Drawing for the job (mm, zero at the part's lowest x, y, z). A direction names the side the tool comes from. Give positions to 0.01 mm unless a question says otherwise; leave off trailing zeros. Write each loop counter-clockwise with the first axis right and the second up, starting at its lowest first coordinate (ties: lowest second). Pieces come first, ordered by that corner, then holes. Notation, with made-up numbers: (35.25, -38) - (90.25, -38) arc R31 cw to (90.25, -7) - close; hole circle Ø1 at (78, -19.75). An arc over 180 degrees is marked (long way). Use CSV: the item, a comma, the result in double quotes.
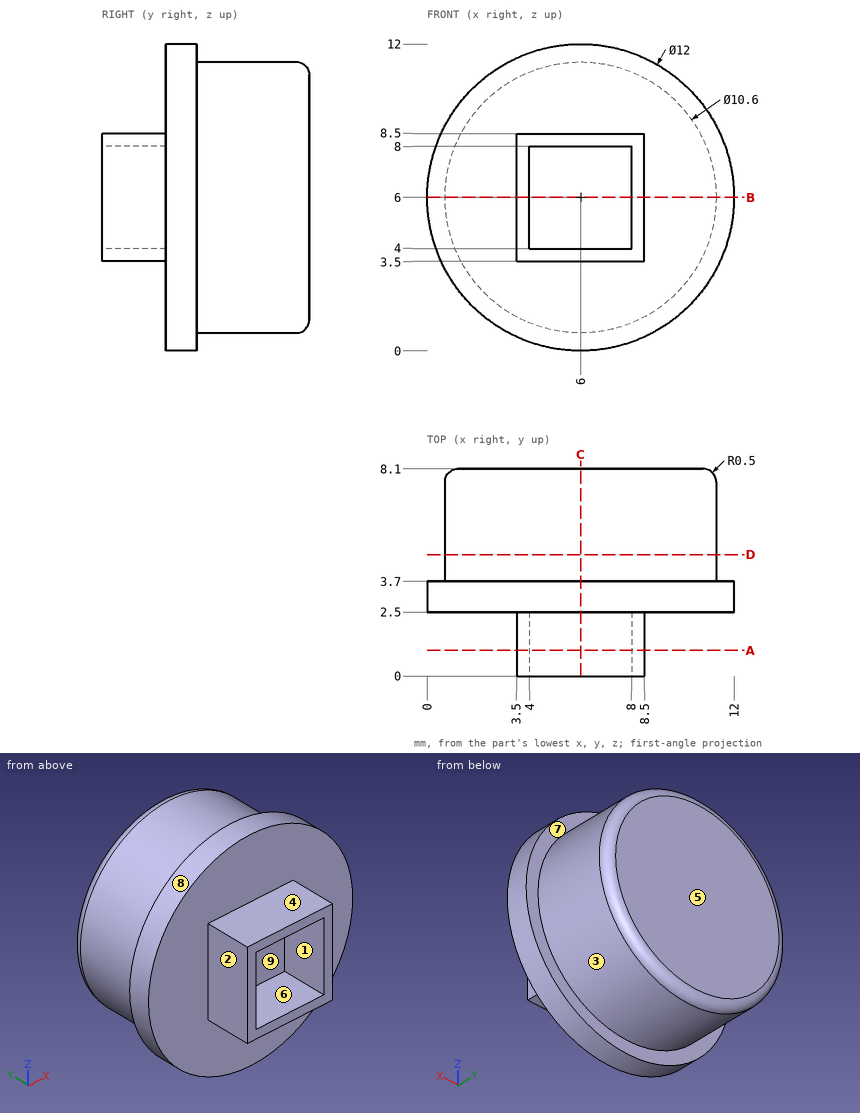
(1) Pull direction Z, two halves, no side cores. Call the marked faces 6, 7, 8 and 9: released by +Z, released by -Z, zero draft, split by the parting line, or undercut.
Checked values:
face 6,"undercut"
face 7,"zero draft"
face 8,"split by the parting line"
face 9,"undercut"
(2) Flat gauge pins, fed straight in: P1, Ø2, axis at x = 5, y = 2, coming from the -Z side; P2, Ø0.8, axis at x = 6, y = 1, coming from the +Z side; P3, Ø2, axis at y = 0.5, z = 5.5, coming from the +X side. Where does each tip first touch, or does it go through?
Checked values:
P1,"stops at z = 0"
P2,"stops at z = 8.5"
P3,"stops at x = 8.5"
(3) Saw through at D-D, the plane y = 4.75. List the corners of the cut face in (x, z).
Checked values:
outline,"circle Ø10.6 at (6, 6)"
(4) Saw through at B-B, the plane z = 6. List the corners of the cut face in (x, y).
Checked values:
outline,"(0, 2.5) - (3.5, 2.5) - (3.5, 0) - (4, 0) - (4, 2.5) - (8, 2.5) - (8, 0) - (8.5, 0) - (8.5, 2.5) - (12, 2.5) - (12, 3.7) - (11.3, 3.7) - (11.3, 7.6) arc R0.5 ccw to (10.8, 8.1) - (1.2, 8.1) arc R0.5 ccw to (0.7, 7.6) - (0.7, 3.7) - (0, 3.7) - close"
(5) 3-axis set-ups, long thin cutter, end or side, ignore diameter. For the marked faces 1, 2, 3, 4 and 5: which of +Z, -Z, +X, -X, +Y, -Y reach the whole face in a straight line?
Checked values:
face 1,"-Y"
face 2,"+Z, -Z, -X, -Y"
face 3,"+Y"
face 4,"+Z, +X, -X, -Y"
face 5,"+Z, -Z, +X, -X, +Y"
(6) Wall check: probe 1 along X at (y, z) = (2, 6.5); probe 2 along Y at (x, z) = (6.75, 3); probe 3 along Z at (x, y) = (6, 6.75). Give the ranges that are in metal, low to high. Write a range as [from, to].
Checked values:
probe 1,"x = [3.5, 4], [8, 8.5]"
probe 2,"y = [2.5, 8.1]"
probe 3,"z = [0.7, 11.3]"
(7) Saw through at C-C, the plane x = 6. List the corners of the cut face in (y, z).
Checked values:
outline,"(0, 3.5) - (2.5, 3.5) - (2.5, 0) - (3.7, 0) - (3.7, 0.7) - (7.6, 0.7) arc R0.5 ccw to (8.1, 1.2) - (8.1, 10.8) arc R0.5 ccw to (7.6, 11.3) - (3.7, 11.3) - (3.7, 12) - (2.5, 12) - (2.5, 8.5) - (0, 8.5) - (0, 8) - (2.5, 8) - (2.5, 4) - (0, 4) - close"
(8) Saw through at A-A, the plane y = 1. List the corners of the cut face in (x, z), then the cut area to 3 significant figures.
Checked values:
outline,"(3.5, 3.5) - (8.5, 3.5) - (8.5, 8.5) - (3.5, 8.5) - close; hole (4, 4) - (8, 4) - (8, 8) - (4, 8) - close"
area,"9.00 mm^2"
